```python
from build123d import *

# Parameters (mm, degrees)
F0_W     = 50
F0_H     = 150
F0_R     = 5
F1_DEPTH = 50
F3_D     = 5
F3_DEPTH = 15
F3_TIP   = 1.5021515476


with BuildPart() as f1:
    # F0 (on Front) → F1 (new body)
    with BuildSketch(Plane.XZ):
        Rectangle(F0_W, F0_H)
        with Locations((0, 50)):
            Circle(F0_R, mode=Mode.SUBTRACT)
    extrude(amount=F1_DEPTH)

    # F3
    with Locations(Plane(origin=(0, 0, -75), x_dir=(1, 0, 0), z_dir=(0, 0, -1))):
        with Locations((12.5, 37.5), (12.5, 12.5), (-12.5, 12.5), (-12.5, 37.5)):
            Hole(F3_D / 2, depth=F3_DEPTH)
            with Locations((0, 0, -(F3_DEPTH + F3_TIP / 2))):  # 118° drill point
                Cone(0, F3_D / 2, F3_TIP, mode=Mode.SUBTRACT)


solid = f1.part
```
Geometry: final body of the model. Coordinates: model frame, mm. A direction names the side the tool comes from. Give positions to 0.01 mm unless a question says otherwise; leave off trailing zeros. Loops run counter-clockwise (first coordinate to the right, second up) from the corner with the lowest first, then second, coordinate; pieces in that order, holes last. Notation, with made-up numbers: (89, 22.5) -> (100, 22.5) arc R25 cw to (100, 37.5) -> close; hole circle Ø5 at (44.25, 65). An arc over 180 degrees is marked (long way). Return JSON: item names as keys, results as strings.
Item 1: Section B-B, the plane z = 50. Output: boundary loops of the cut face in (x, y).
Filled in:
{"outline": "(-25, -50) -> (-5, -50) -> (-5, 0) -> (-25, 0) -> close; (5, -50) -> (25, -50) -> (25, 0) -> (5, 0) -> close"}
Item 2: Section A-A, the plane x = 0. Output: boundary loops of the cut face in (y, z), plus the area to 3 significant figures.
Filled in:
{"outline": "(-50, -75) -> (0, -75) -> (0, 45) -> (-50, 45) -> close; (-50, 55) -> (0, 55) -> (0, 75) -> (-50, 75) -> close", "area": "7,000 mm^2"}
Item 3: Section C-C, the plane z = -66. Output: boundary loops of the cut face in (x, y).
Filled in:
{"outline": "(-25, -50) -> (25, -50) -> (25, 0) -> (-25, 0) -> close; hole circle Ø5 at (-12.5, -37.5); hole circle Ø5 at (-12.5, -12.5); hole circle Ø5 at (12.5, -37.5); hole circle Ø5 at (12.5, -12.5)"}
Item 4: Pin query (flat end, axial travel): P1, Ø6.5, axis at x = 12.5, y = -37.5, coming from the -Z side. Return the tip coordinate at first contact, or that it passes through.
Filled in:
{"P1": "z = -75"}
Item 5: Line query: line 1 (X direction, y = -12.5, z = -63.75); line 2 (Z direction, x = 0, y = -2.5); line 3 (Y direction, x = 12.5, z = -68.5). Output: solid intervals per line, ascending.
Filled in:
{"line 1": "-25 to -15, -10 to 10, 15 to 25", "line 2": "-75 to 45, 55 to 75", "line 3": "-50 to -40, -35 to -15, -10 to 0"}
Item 6: Mould query, pull axis X, two halves, no side actions, for faces 1 (the flat face through (25, -25, -1)), 2 (the flat face through (0, 0, 1)), 3 (the cylindrical face through (-11.96, -35.06, -67.4)). Classes: released by +X, released by -X, zero draft, split by the parting line, or undercut.
Filled in:
{"face 1": "released by +X", "face 2": "zero draft", "face 3": "undercut"}
Item 7: Access query for faces 4 (the cylindrical face through (-0.651, -24.65, 54.957)), 5 (the cylindrical face through (-11.96, -10.06, -67.4)). Directions: +Z, -Z, +X, -X, +Y, -Y. A direction counts if a zero-diameter tool reaches every point of the face in a straight line with its end or side. Return the directions, or none.
Filled in:
{"face 4": "+Y, -Y", "face 5": "-Z"}
